For this review, take the finished solid that the model builds, in its own axes (mm). A direction names the side the tool comes from. Round coordinates to 2 decimals unless told otherwise and drop trailing zeros. Order: outer loops, then holes, each group sorted by start corner. A loop starts at its lowest first (then second) coordinate and runs counter-clockwise, first axis right, second up. Notation, with made-up numbers: (-27, 86) - (12, 86) arc R22 ccw to (12, 114) - close; hole circle Ø6 at (9.25, -15.5). An arc over 180 degrees is marked (long way). One line per question, with ' | ' between items.
```python
from build123d import *

# Parameters (mm, degrees)
SKETCH1_W           = 40
SKETCH1_H           = 20
BOSS_EXTRUDE1_DEPTH = 40
BOSS_EXTRUDE2_START = 40
SKETCH2_R           = 3
BOSS_EXTRUDE2_DEPTH = 4
BOSS_EXTRUDE3_START = 27.75
SKETCH3_W           = 56
SKETCH3_H           = 20
SKETCH3_R           = 2.1
BOSS_EXTRUDE3_DEPTH = 2.7


with BuildPart() as part:
    # Sketch1 → Boss-Extrude1 (new body)
    with BuildSketch(Plane.XY):
        Rectangle(SKETCH1_W, SKETCH1_H)
    extrude(amount=BOSS_EXTRUDE1_DEPTH)

    # Sketch2 → Boss-Extrude2 (add)
    with BuildSketch(Plane.XY.offset(BOSS_EXTRUDE2_START)):
        with Locations(Location((10, 0, 0), (0, 0, 180))):
            Circle(SKETCH2_R)
    extrude(amount=BOSS_EXTRUDE2_DEPTH)

    # Sketch3 → Boss-Extrude3 (add)
    with BuildSketch(Plane.XY.offset(BOSS_EXTRUDE3_START)):
        Rectangle(SKETCH3_W, SKETCH3_H)
        with Locations(Location((-24, 5, 0), (0, 0, 180))):
            Circle(SKETCH3_R, mode=Mode.SUBTRACT)
        with Locations(Location((-24, -5, 0), (0, 0, 180))):
            Circle(SKETCH3_R, mode=Mode.SUBTRACT)
        with Locations(Location((24, -5, 0), (0, 0, 180))):
            Circle(SKETCH3_R, mode=Mode.SUBTRACT)
        with Locations(Location((24, 5, 0), (0, 0, 180))):
            Circle(SKETCH3_R, mode=Mode.SUBTRACT)
    extrude(amount=BOSS_EXTRUDE3_DEPTH)


solid = part.part
```
(1) Insertion check: pin 1 (8 mm diameter, centred on y = 6.5, z = 14.5, fed in from -X); pin 2 (4 mm diameter, centred on x = -24, y = -5, fed in from +Z); pin 3 (5 mm diameter, centred on x = 24, y = -5, fed in from -Z); pin 4 (4 mm diameter, centred on x = 25.5, y = 1.5, fed in from +Z). Each pin has a flat end and moves straight along its axis. Give the tip position at first contact, or say it passes through.
Output values:
pin 1: x = -20 | pin 2: through | pin 3: z = 27.75 | pin 4: z = 30.45
(2) We need section A-A on y = 5. State the section outline as (x, z) points, plus the area to 3 significant figures.
Output values:
outline: (-28, 27.75) - (-26.1, 27.75) - (-26.1, 30.45) - (-28, 30.45) - close; (-21.9, 27.75) - (-20, 27.75) - (-20, 0) - (20, 0) - (20, 27.75) - (21.9, 27.75) - (21.9, 30.45) - (20, 30.45) - (20, 40) - (-20, 40) - (-20, 30.45) - (-21.9, 30.45) - close; (26.1, 27.75) - (28, 27.75) - (28, 30.45) - (26.1, 30.45) - close | area: 1,620 mm^2
(3) For faces 1 (the flat face through (-24, 0, 30.45)), 2 (the flat face through (20, 0, 14)), 3 (the flat face through (24, 0, 30.45)), 4 (the flat face through (-20, 0, 14)), 5 (the cylindrical face through (-24.969, 6.863, 29.081)), list the 3-axis set-ups (+Z, -Z, +X, -X, +Y, -Y) from which the entire face can be reached by the end or side of a thin tool; tool diameter is ignored.
Output values:
face 1: +Z, -X, +Y, -Y | face 2: -Z, +X, +Y, -Y | face 3: +Z, +X, +Y, -Y | face 4: -Z, -X, +Y, -Y | face 5: +Z, -Z
(4) Mouldability with a two-part tool opening along Y and no side actions: class faces 6 (the cylindrical face through (-26.003, -5.631, 29.081)), 7 (the flat face through (0, 0, 0)), 8 (the cylindrical face through (13, 0, 42)) as released by +Y, released by -Y, zero draft, split by the parting line, or undercut.
Output values:
face 6: undercut | face 7: zero draft | face 8: split by the parting line
(5) We need section D-D on x = 8.5. State the section outline as (y, z) points, plus the area to 3 significant figures.
Output values:
outline: (-10, 0) - (10, 0) - (10, 40) - (2.6, 40) - (2.6, 44) - (-2.6, 44) - (-2.6, 40) - (-10, 40) - close | area: 821 mm^2
(6) We need section B-B on x = -24. State the section outline as (y, z) points.
Output values:
outline: (-10, 27.75) - (-7.1, 27.75) - (-7.1, 30.45) - (-10, 30.45) - close; (-2.9, 27.75) - (2.9, 27.75) - (2.9, 30.45) - (-2.9, 30.45) - close; (7.1, 27.75) - (10, 27.75) - (10, 30.45) - (7.1, 30.45) - close
(7) We need section C-C on y = 7.75. State the section outline as (x, z) points, plus the area to 3 significant figures.
Output values:
outline: (-28, 27.75) - (-20, 27.75) - (-20, 0) - (20, 0) - (20, 27.75) - (28, 27.75) - (28, 30.45) - (20, 30.45) - (20, 40) - (-20, 40) - (-20, 30.45) - (-28, 30.45) - close | area: 1,640 mm^2
(8) For probe 1 along X at (y, z) = (5, 28.6); probe 2 along Y at (x, z) = (24, 29.35); probe 3 along Z at (x, y) = (24.5, -2.5), list the stretches that pass through material, from the lowest coordinate up. Write a range as [from, to].
Output values:
probe 1: [-28, -26.1], [-21.9, 21.9], [26.1, 28] | probe 2: [-10, -7.1], [-2.9, 2.9], [7.1, 10] | probe 3: [27.75, 30.45]
